For this review, take the finished solid that the model builds, in its own axes (mm). Face numbers are marked on the shaded views. A direction names the side the tool comes from. Coordinates: 2 decimals unless noted, no trailing zeros. Order: outer loops, then holes, each group sorted by start corner. A loop starts at its lowest first (then second) coordinate and runs counter-clockwise, first axis right, second up. Notation, with made-up numbers: (-37.75, 5) -> (-10.75, 5) arc R13 cw to (-10.75, 21) -> close; hole circle Ø5 at (76, 11.25). An arc over 180 degrees is marked (long way). Write item = value, one per line. Start each with the question number.
1) Consider section A-A on x = -15.5. Give the boundary of the cut face in (y, z).
2) Consider section B-B on z = 23.3. Give the boundary of the cut face in (x, y).
3) Consider section D-D on z = 7.8. Give the boundary of the cut face in (x, y), and give its area (3 significant figures).
4) Consider section C-C on y = 4. Give the boundary of the cut face in (x, z).
5) Insertion check: pin 1 Ø10 at (x, y) = (-12, 12.5) entering from +Z; pin 2 Ø2.5 at (x, y) = (-26.8, 35) entering from +Z; pin 3 Ø6 at (y, z) = (6, 26.5) entering from +X; pin 4 Ø5.5 at (x, z) = (15.5, 38.8) entering from +Y. Each pin has a flat end and moves straight along its axis. Give the tip position at first contact, or say it passes through.
6) Wall thickness on probe 1 along Z at (x, y) = (15.5, 1.35); probe 2 along X at (y, z) = (35, 1.05); probe 3 along Y at (x, z) = (26, 1): over which ranges is each line inside the solid? List them lowest first. Write a range as [from, to].
7) Machinability: for the marked faces 4, 5 and 6, which of the approach directions +Z, -Z, +X, -X, +Y, -Y give a long, thin tool a straight path to every point of the face, cutting with its end or side? Answer none if there is none.
8) Draft analysis for pull direction X (two halves, no side actions). For the marked faces 1, 2 and 3, state which applies: +X half, -X half, draft (parallel to the pull), parting line (faces both ways), or undercut.
from build123d import *

# Parameters (mm, degrees)
PAD_DEPTH       = 31
POCKET_DEPTH    = 42
SKETCH002_R     = 1.7
POCKET001_DEPTH = 44.001
SKETCH003_R     = 1.7
SKETCH003_R_2   = 11.3
POCKET002_DEPTH = 40.001
FILLET_R        = 2.5


with BuildPart() as part:
    # Sketch → Pad (new body, symmetric)
    with BuildSketch(Plane.YZ):
        Polygon((0, 44), (2, 44), (40, 2), (40, 0), (0, 0), align=None)
    extrude(amount=PAD_DEPTH, both=True)

    # Sketch001 → Pocket (cut)
    with BuildSketch(Plane.XY.offset(44)):
        Polygon((-32, 42), (-32, -1), (-23.3, -1), (-23.3, 41), (-21.3, 41), (-21.3, 2), (21.3, 2), (21.3, 41), (23.3, 41), (23.3, -1), (32, -1), (32, 42), align=None)
    extrude(amount=-POCKET_DEPTH, mode=Mode.SUBTRACT)

    # Sketch002 → Pocket001 (cut, through all)
    with BuildSketch(Plane.XY):
        with Locations((-26.8, 35)):
            Circle(SKETCH002_R)
        with Locations((-26.8, 20)):
            Circle(SKETCH002_R)
        with Locations((-26.8, 5)):
            Circle(SKETCH002_R)
        with Locations((26.8, 35)):
            Circle(SKETCH002_R)
        with Locations((26.8, 20)):
            Circle(SKETCH002_R)
        with Locations((26.8, 5)):
            Circle(SKETCH002_R)
    extrude(amount=POCKET001_DEPTH, mode=Mode.SUBTRACT)

    # Sketch003 → Pocket002 (cut, through all)
    with BuildSketch(Plane.XZ):
        with Locations((-15.5, 38.8)):
            Circle(SKETCH003_R)
        with Locations((15.5, 38.8)):
            Circle(SKETCH003_R)
        with Locations((15.5, 7.8)):
            Circle(SKETCH003_R)
        with Locations((-15.5, 7.8)):
            Circle(SKETCH003_R)
        with Locations((0, 23.3)):
            Circle(SKETCH003_R_2)
    extrude(amount=-POCKET002_DEPTH, mode=Mode.SUBTRACT)

    # Fillet
    fillet_edges = [part.edges().sort_by_distance(p)[0] for p in [
        (31, 40, 1),
        (31, 0, 1),
        (-31, 40, 1),
        (-31, 0, 1),
    ]]
    fillet(fillet_edges, radius=FILLET_R)


solid = part.part
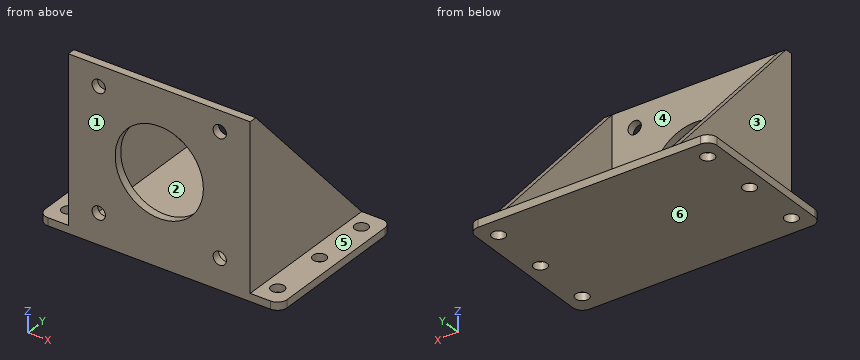
Answer sheet:
q1.outline = (0, 0) -> (40, 0) -> (40, 2) -> (2, 2) -> (2, 6.1) -> (0, 6.1) -> close; (0, 9.5) -> (2, 9.5) -> (2, 37.1) -> (0, 37.1) -> close; (0, 40.5) -> (2, 40.5) -> (2, 44) -> (0, 44) -> close
q2.outline = (-23.3, 0) -> (-11.3, 0) -> (-11.3, 2) -> (-21.3, 2) -> (-21.3, 20.73) -> (-23.3, 20.73) -> close; (11.3, 0) -> (23.3, 0) -> (23.3, 20.73) -> (21.3, 20.73) -> (21.3, 2) -> (11.3, 2) -> close
q3.outline = (-23.3, 0) -> (-17.2, 0) -> (-17.2, 2) -> (-21.3, 2) -> (-21.3, 34.75) -> (-23.3, 34.75) -> close; (-13.8, 0) -> (13.8, 0) -> (13.8, 2) -> (-13.8, 2) -> close; (17.2, 0) -> (23.3, 0) -> (23.3, 34.75) -> (21.3, 34.75) -> (21.3, 2) -> (17.2, 2) -> close
q3.area = 211 mm2
q4.outline = (-31, 0) -> (-28.17, 0) -> (-28.17, 2) -> (-31, 2) -> close; (-25.43, 0) -> (25.43, 0) -> (25.43, 2) -> (23.3, 2) -> (23.3, 41.79) -> (21.3, 41.79) -> (21.3, 2) -> (-21.3, 2) -> (-21.3, 41.79) -> (-23.3, 41.79) -> (-23.3, 2) -> (-25.43, 2) -> close; (28.17, 0) -> (31, 0) -> (31, 2) -> (28.17, 2) -> close
q5.pin_1 = 2
q5.pin_2 = through
q5.pin_3 = 23.3
q5.pin_4 = 2
q6.probe_1 = [0, 6.1], [9.5, 37.1], [40.5, 44]
q6.probe_2 = [-31, -28.5], [-25.1, 25.1], [28.5, 31]
q6.probe_3 = [0, 3.5], [6.5, 18.5], [21.5, 33.5], [36.5, 40]
q7.face_4 = +Z, +Y
q7.face_5 = +Z, +X, +Y, -Y
q7.face_6 = -Z, +X, -X, +Y, -Y
q8.face_1 = draft
q8.face_2 = undercut
q8.face_3 = -X half
